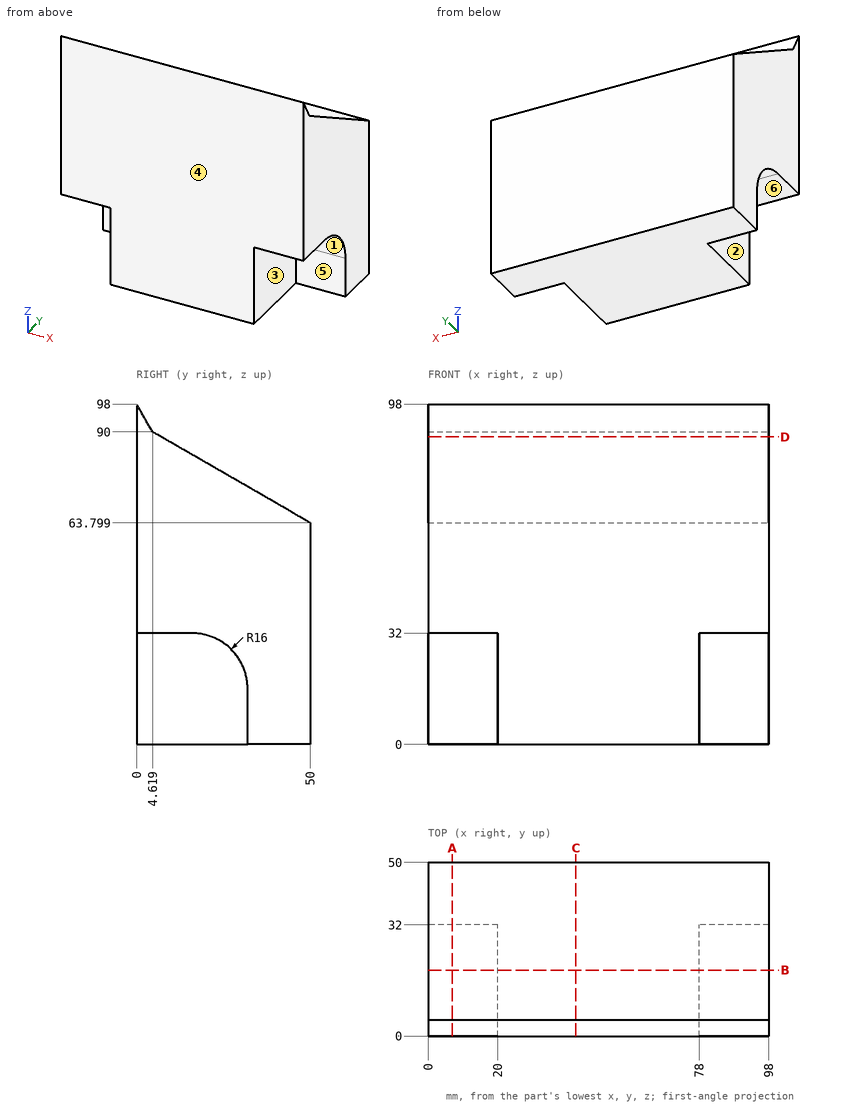
Print and shaded views of the part. All mm, measured from the part's lowest x, y and z. A direction names the side the tool comes from. Round coordinates to 2 decimals unless told otherwise and drop trailing zeros. Write each loop counter-clockwise with the first axis right and the second up, starting at its lowest first coordinate (ties: lowest second). Pieces come first, ordered by that corner, then holes.
(1) Slice it at D-D, the plane z = 88.5. Write the cut outline in (x, y), and give its area (3 significant figures).
(2) Drop flat-ended pins along their axis: P1, Ø3, axis at x = 36, y = 15.5, coming from the +Z side; P2, Ø3, axis at x = 11.5, y = 19, coming from the +Z side; P3, Ø6, axis at y = 26, z = 15.5, coming from the -X side. Give the stop position or say it passes through.
(3) Slice it at C-C, the plane x = 42.5. Write the cut outline in (y, z), and give its area (3 significant figures).
(4) Mould opens along X. For the marked faces 1, 2 and 3 say: pulls with the +X half, pulls with the -X half, needs draft (parallel to the pull), parting line crosses it, or undercut.
(5) 3-axis set-ups, long thin cutter, end or side, ignore diameter. For the marked faces 4, 5 and 6: which of +Z, -Z, +X, -X, +Y, -Y reach the whole face in a straight line?
(6) Slice it at A-A, the plane x = 7. Write the cut outline in (y, z).
(7) Probe line 1 along X through (y, z) = (23, 22); line 2 along Y through (x, z) = (93.5, 9.5); line 3 along Y through (x, z) = (87, 23). List the from-to ranges inside material, lowest first.
(8) Slice it at B-B, the plane y = 19. Write the cut outline in (x, z), and give its area (3 significant figures).
From the geometry:
1. outline: (0, 0) - (98, 0) - (98, 7.22) - (0, 7.22) - close
1. area: 707 mm2
2. P1: stops at z = 84.58
2. P2: stops at z = 82.56
2. P3: stops at x = 20
3. outline: (0, 0) - (50, 0) - (50, 63.8) - (4.62, 90) - (0, 98) - close
3. area: 3,920 mm2
4. face 1: needs draft
4. face 2: pulls with the -X half
4. face 3: pulls with the +X half
5. face 4: +Z, -Z, +X, -X, -Y
5. face 5: -Z, +X, -Y
5. face 6: -Z, -X, -Y
6. outline: (0, 32) - (16, 32) arc R16 cw to (32, 16) - (32, 0) - (50, 0) - (50, 63.8) - (4.62, 90) - (0, 98) - close
7. line 1: x = 20 to 78
7. line 2: y = 32 to 50
7. line 3: y = 30.39 to 50
8. outline: (0, 31.72) - (20, 31.72) - (20, 0) - (78, 0) - (78, 31.72) - (98, 31.72) - (98, 81.7) - (0, 81.7) - close
8. area: 6,740 mm2
